Read the model definition and answer for the solid it produces. Units are mm, in the model's axes. Give positions to 0.01 mm unless a question says otherwise; leave off trailing zeros. Order: outer loops, then holes, each group sorted by start corner. A loop starts at its lowest first (then second) coordinate and runs counter-clockwise, first axis right, second up. Notation, with made-up numbers: (68.25, -14) -> (113.25, -14) arc R23 ccw to (113.25, 19) -> close; hole circle Ø11 at (28, -28). An arc over 180 degrees is marked (long way). One line per item, written item: value. Start each with the question number.
from build123d import *

# Parameters (mm, degrees)
ESQUISSE1_W                  = 233
ESQUISSE1_H                  = 300
BOSS_EXTRU_1_DEPTH           = 4.2
ESQUISSE2_R                  = 2.55
ESQUISSE2_W                  = 102.8
ESQUISSE2_H                  = 40.2
ENL_V_MAT_EXTRU_1_DEPTH      = 1
ENL_V_MAT_EXTRU_1_DEPTH_BACK = 5.2


with BuildPart() as part:
    # Esquisse1 → Boss.-Extru.1 (new body)
    with BuildSketch(Plane.XY):
        with Locations((-45.332061069, 23.536895674)):
            Rectangle(ESQUISSE1_W, ESQUISSE1_H)
    extrude(amount=BOSS_EXTRU_1_DEPTH)

    # Esquisse2 → Enlèv. mat.-Extru.1 (cut, two sides)
    with BuildSketch(Plane.XY.offset(4.2)) as enl_v_mat_extru_1_sk:
        with Locations((-102.632061069, 131.426895674)):
            Circle(ESQUISSE2_R)
        with Locations((11.967938931, 131.426895674)):
            Circle(ESQUISSE2_R)
        with Locations((-102.632061069, 81.426895674)):
            Circle(ESQUISSE2_R)
        with Locations((11.967938931, 81.426895674)):
            Circle(ESQUISSE2_R)
        with Locations((-102.632061069, 31.426895674)):
            Circle(ESQUISSE2_R)
        with Locations((11.967938931, 31.426895674)):
            Circle(ESQUISSE2_R)
        with Locations((-102.632061069, -18.573104326)):
            Circle(ESQUISSE2_R)
        with Locations((11.967938931, -18.573104326)):
            Circle(ESQUISSE2_R)
        with Locations((-45.332061069, -22.123104326)):
            Rectangle(ESQUISSE2_W, ESQUISSE2_H)
        with Locations((-45.332061069, 27.876895674)):
            Rectangle(ESQUISSE2_W, ESQUISSE2_H)
        with Locations((-45.332061069, 77.876895674)):
            Rectangle(ESQUISSE2_W, ESQUISSE2_H)
        with Locations((-45.332061069, 127.876895674)):
            Rectangle(ESQUISSE2_W, ESQUISSE2_H)
    extrude(amount=ENL_V_MAT_EXTRU_1_DEPTH, mode=Mode.SUBTRACT)
    extrude(enl_v_mat_extru_1_sk.sketch, amount=-ENL_V_MAT_EXTRU_1_DEPTH_BACK, mode=Mode.SUBTRACT)


solid = part.part
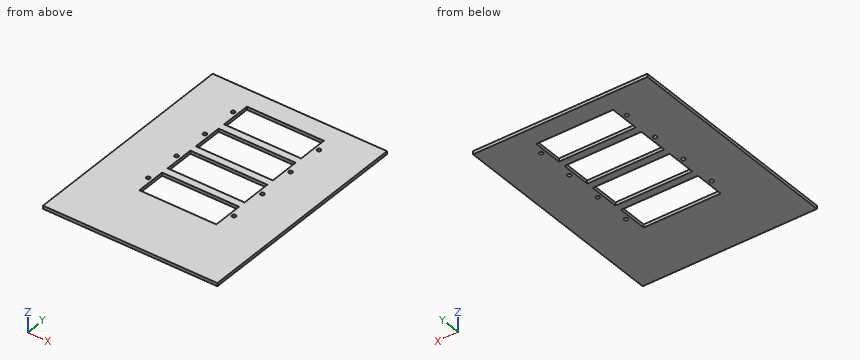
Item 1: Find the intervals of material crossed by line 1 (Y direction, x = -27, z = 2.95); line 2 (X direction, y = 38.5, z = 1); line 3 (X direction, y = -20, z = 0.75), in increasing order. Write a range as from..to.
Item 2: Find section A-A on x = -72. Write down the section's boundary in (y, z).
Item 3: Find section B-B on y = 112. Write down the section's boundary in (x, z), then the cut area to 3 significant figures.
Item 4: A flat-ended cylindrical pin translates along its axis: pin 1 (4.5 mm diameter, centred on x = -102.63, y = 131.43, fed in from -Z). Find the tip coordinate at first contact, or state that the pin passes through.
Item 5: Find section C-C on z = 1.9. Count the separate pieces of the cut face and the enclosed holes in it, then the cut area to 3 significant figures.
Checks:
1. line 1: -126.46..-42.22, -2.02..7.78, 47.98..57.78, 97.98..107.78, 147.98..173.54
1. line 2: -161.83..-96.73, 6.07..71.17
1. line 3: -161.83..-104.75, -100.52..-96.73, 6.07..9.85, 14.08..71.17
2. outline: (-126.46, 0) -> (-42.22, 0) -> (-42.22, 4.2) -> (-126.46, 4.2) -> close; (-2.02, 0) -> (7.78, 0) -> (7.78, 4.2) -> (-2.02, 4.2) -> close; (47.98, 0) -> (57.78, 0) -> (57.78, 4.2) -> (47.98, 4.2) -> close; (97.98, 0) -> (107.78, 0) -> (107.78, 4.2) -> (97.98, 4.2) -> close; (147.98, 0) -> (173.54, 0) -> (173.54, 4.2) -> (147.98, 4.2) -> close
3. outline: (-161.83, 0) -> (-96.73, 0) -> (-96.73, 4.2) -> (-161.83, 4.2) -> close; (6.07, 0) -> (71.17, 0) -> (71.17, 4.2) -> (6.07, 4.2) -> close
3. area: 547 mm2
4. pin 1: through
5. separate pieces: 1
5. enclosed holes: 12
5. area: 53,200 mm2
